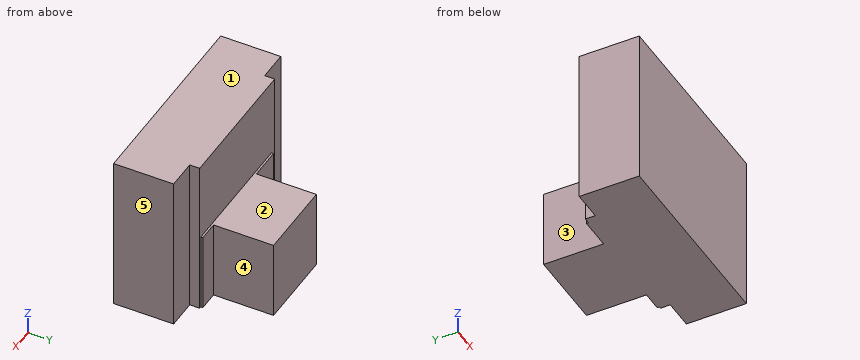
```python
from build123d import *

# Parameters (mm, degrees)
SKETCH_1_W          = 100
SKETCH_1_H          = 80
EXTRUDE_1_DEPTH     = 35
SKETCH_2_W          = 66
SKETCH_2_H          = 40
EXTRUDE_2_DEPTH     = 1
SKETCH_3_W          = 40
SKETCH_3_H          = 40
EXTRUDE_3_DEPTH     = 30
SKETCH_4_W          = 15
SKETCH_4_H          = 80
CUT_EXTRUDE_1_DEPTH = 5


with BuildPart() as part:
    # 草图1 → 凸台-拉伸1 (new body)
    with BuildSketch(Plane(origin=(0, 0, 0), x_dir=(1, 0, 0), z_dir=(0, 1, 0))):
        with Locations((50, 40)):
            Rectangle(SKETCH_1_W, SKETCH_1_H)
    extrude(amount=EXTRUDE_1_DEPTH)

    # 草图2 → 凸台-拉伸2 (add)
    with BuildSketch(Plane(origin=(0, 35, 0), x_dir=(1, 0, 0), z_dir=(0, 1, 0))):
        with Locations((51, 60)):
            Rectangle(SKETCH_2_W, SKETCH_2_H)
    extrude(amount=EXTRUDE_2_DEPTH)

    # 草图3 → 凸台-拉伸3 (add)
    with BuildSketch(Plane(origin=(0, 36, 0), x_dir=(1, 0, 0), z_dir=(0, 1, 0))):
        with Locations((54, 60)):
            Rectangle(SKETCH_3_W, SKETCH_3_H)
    extrude(amount=EXTRUDE_3_DEPTH)

    # 草图4 → 切除-拉伸1 (cut)
    with BuildSketch(Plane(origin=(0, 35, 0), x_dir=(1, 0, 0), z_dir=(0, 1, 0))):
        with Locations((7.5, 40)):
            Rectangle(SKETCH_4_W, SKETCH_4_H)
        with Locations((92.5, 40)):
            Rectangle(SKETCH_4_W, SKETCH_4_H)
    extrude(amount=-CUT_EXTRUDE_1_DEPTH, mode=Mode.SUBTRACT)


solid = part.part
```
Can you work these out from the model? Positions are in its coordinate system, mm. Face numbers are marked on the shaded views. A direction names the side the tool comes from. Coordinates: 2 decimals unless noted, no trailing zeros. Loops run counter-clockwise (first coordinate to the right, second up) from the corner with the lowest first, then second, coordinate; pieces in that order, holes last.
1) I need wall thicknesses on probe 1 along Y at (x, z) = (19, -68); probe 2 along Z at (x, y) = (36.5, 59); probe 3 along Y at (x, z) = (92, -48.5). Which ranges of each line are inside material? Lowest first, please.
2) Imagine slicing it at A-A on z = -65.5. List the corners of the cut face in (x, y) for me.
3) Which directions (+Z, -Z, +X, -X, +Y, -Y) give clear straight access to the entire face, cutting with the end or side of a thin tool? Please do the marked faces 1, 2, 3, 4 and 5.
4) Imagine slicing it at B-B on x = 77.5. List the corners of the cut face in (y, z) for me, plus the area to 3 significant figures.
5) Imagine slicing it at D-D on z = -8. List the corners of the cut face in (x, y) for me, plus the area to 3 significant figures.
6) For pin 1 (15.5 mm diameter, centred on x = 49.5, y = 47.5, fed in from +Z); pin 2 (16.5 mm diameter, centred on x = 4.5, z = -47, fed in from +Y); pin 3 (5 mm diameter, centred on x = 79.5, z = -58, fed in from +Y), each with a flat end and sliding along its axis, tell me the tip position at first contact or that it passes through.
7) Imagine slicing it at C-C on y = 46. List the corners of the cut face in (x, z) for me.
Completed:
1. probe 1: y = 0 to 36
1. probe 2: z = -80 to -40
1. probe 3: y = 0 to 30
2. outline: (0, 0) - (100, 0) - (100, 30) - (85, 30) - (85, 35) - (84, 35) - (84, 36) - (74, 36) - (74, 66) - (34, 66) - (34, 36) - (18, 36) - (18, 35) - (15, 35) - (15, 30) - (0, 30) - close
3. face 1: +Z, +X, -X, +Y, -Y
3. face 2: +Z, +X, -X, +Y
3. face 3: +Z, -Z, -X, +Y
3. face 4: +Z, -Z, +X, +Y
3. face 5: +Z, -Z, +X, +Y, -Y
4. outline: (0, -80) - (36, -80) - (36, -40) - (35, -40) - (35, 0) - (0, 0) - close
4. area: 2,840 mm2
5. outline: (0, 0) - (100, 0) - (100, 30) - (85, 30) - (85, 35) - (15, 35) - (15, 30) - (0, 30) - close
5. area: 3,350 mm2
6. pin 1: stops at z = -40
6. pin 2: stops at y = 30
6. pin 3: stops at y = 36
7. outline: (34, -80) - (74, -80) - (74, -40) - (34, -40) - close
